from build123d import *

# Parameters (mm, degrees)
BOSS_EXTRU_1_DEPTH      = 10
ENL_V_MAT_EXTRU_4_DEPTH = 60
BOSS_EXTRU_2_DEPTH      = 40


with BuildPart() as part:
    # Esquisse1 → Boss.-Extru.1 (new body)
    with BuildSketch(Plane.XY):
        Polygon((-50, -37.5), (50, -37.5), (50, 37.5), (10, 37.5), (10, 33.5), (-10, 33.5), (-10, 37.5), (-50, 37.5), align=None)
    extrude(amount=BOSS_EXTRU_1_DEPTH)

    # Esquisse4 → Enl_v. mat.-Extru.4 (cut)
    with BuildSketch(Plane(origin=(50, 0, 0), x_dir=(0, 0, -1), z_dir=(1, 0, 0))):
        Polygon((-10, 33.5), (0, 23.5), (0, 33.5), align=None)
    extrude(amount=-ENL_V_MAT_EXTRU_4_DEPTH, mode=Mode.SUBTRACT)


with BuildPart() as enl_v_mat_extru_4_piece_1:
    # of the separate pieces the step leaves, piece 1, a body of its own (enl_v_mat_extru_4_pieces)
    add(part.part.solids().sort_by_distance((-50, -37.5, 0))[0])



with BuildPart() as enl_v_mat_extru_4_piece_2:
    # of the separate pieces the step leaves, piece 2, a body of its own (enl_v_mat_extru_4_pieces)
    add(part.part.solids().sort_by_distance((10, 37.5, 10))[0])


with BuildPart() as enl_v_mat_extru_4_piece_1_1:
    add(enl_v_mat_extru_4_piece_1.part)

    add(enl_v_mat_extru_4_piece_2.part)  # Boss.-Extru.2 merges Enl_v. mat.-Extru.4 piece 2
    # Esquisse11 → Boss.-Extru.2 (add)
    with BuildSketch(Plane(origin=(50, 0, 0), x_dir=(0, 0, -1), z_dir=(1, 0, 0))):
        Polygon((-10, 33.5), (0, 33.5), (0, 23.5), align=None)
    extrude(amount=-BOSS_EXTRU_2_DEPTH)


solid = enl_v_mat_extru_4_piece_1_1.part
The listing builds one solid part. Answer for the finished solid, in the listing's coordinates (mm). A direction names the side the tool comes from. Round coordinates to 2 decimals unless told otherwise and drop trailing zeros. Write each loop counter-clockwise with the first axis right and the second up, starting at its lowest first coordinate (ties: lowest second). Pieces come first, ordered by that corner, then holes. Notation, with made-up numbers: M -36.75,-23 L -27.75,-23 A15 cw -27.75,-13 Z; hole C -12,22 d9. An arc over 180 degrees is marked long. Write each question's results on one line, items separated by ' | '. Start each with the question number.
(1) Find the intervals of material crossed by line 1 (Y direction, x = 1.5, z = 2.5); line 2 (Y direction, x = 7, z = 5.25), in increasing order.
(2) For faces 4 (the flat face through (0.1, 28.6, 5.1)), 5 (the flat face through (30, 37.5, 5)), determine the directions among +Z, -Z, +X, -X, +Y, -Y from which every point of the face is accessible in a straight line to the end or side of a thin tool.
(3) The part is cut by section A-A, the plane z = 2.5. Write down the section's boundary in (x, y), and give its area (3 significant figures).
(4) Determine the mould class of faces 1 (the flat face through (-30, 37.5, 5)), 2 (the flat face through (-10, 32, 4)), 3 (the flat face through (-50, 1, 5)) for opening direction X: +X half, -X half, draft (parallel to the pull), parting line (faces both ways), or undercut.
(5) This flat-tipped pin is pushed along its axis until it touches: P1, Ø1, axis at x = 28, y = 20, coming from the -Z side. Where does it stop, or does it pass through?
(6) The part is cut by section C-C, the plane x = -3. Write down the section's boundary in (y, z).
(7) The part is cut by section B-B, the plane y = 25. Write down the section's boundary in (x, z), and give its area (3 significant figures).
Worked answers:
1) line 1: y = -37.5 to 26 | line 2: y = -37.5 to 28.75
2) face 4: -Z, +Y | face 5: +Z, -Z, +X, -X, +Y
3) outline: M -50,-37.5 L 50,-37.5 L 50,37.5 L 10,37.5 L 10,26 L -10,26 L -10,37.5 L -50,37.5 Z | area: 7,270 mm²
4) face 1: draft | face 2: undercut | face 3: -X half
5) P1: stops at z = 0
6) outline: M -37.5,0 L 23.5,0 L 33.5,10 L -37.5,10 Z
7) outline: M -50,0 L -10,0 L -10,1.5 L 10,1.5 L 10,0 L 50,0 L 50,10 L -50,10 Z | area: 970 mm²
